from build123d import *

# Parameters (mm, degrees)
SKETCH_1_R          = 1.6
SKETCH_1_R_2        = 3
EXTRUDE_1_DEPTH     = 4
SKETCH_4_R          = 5.25
CUT_EXTRUDE_3_DEPTH = 38.854986461


with BuildPart() as part:
    # 草图1 → 凸台-拉伸1 (new body)
    with BuildSketch(Plane.XY):
        with BuildLine():
            Line((1.833333333, 10.846146269), (31, 5.916079783))
            ThreePointArc((31, 5.916079783), (36, 0), (31, -5.916079783))
            Line((31, -5.916079783), (1.833333333, -10.846146269))
            ThreePointArc((1.833333333, -10.846146269), (-11, 0), (1.833333333, 10.846146269))
        make_face()
        with Locations((0, 7)):
            Circle(SKETCH_1_R, mode=Mode.SUBTRACT)
        with Locations((-7, 0)):
            Circle(SKETCH_1_R, mode=Mode.SUBTRACT)
        with Locations((0, -7)):
            Circle(SKETCH_1_R, mode=Mode.SUBTRACT)
        with Locations((7, 0)):
            Circle(SKETCH_1_R, mode=Mode.SUBTRACT)
        with Locations((30, 0)):
            Circle(SKETCH_1_R_2, mode=Mode.SUBTRACT)
    extrude(amount=EXTRUDE_1_DEPTH)

    # 草图4 → 切除-拉伸3 (cut, through all)
    with BuildSketch(Plane.XY.offset(4)):
        Circle(SKETCH_4_R)
    extrude(amount=-CUT_EXTRUDE_3_DEPTH, mode=Mode.SUBTRACT)


solid = part.part
Design review of the part built by this model. Coordinates are the model's own, in mm. Round coordinates to 2 decimals unless told otherwise and drop trailing zeros. Order: outer loops, then holes, each group sorted by start corner. A loop starts at its lowest first (then second) coordinate and runs counter-clockwise, first axis right, second up. Notation, with made-up numbers: M -32.75,11 L 1.25,11 A15 cw 1.25,31 Z; hole C -36.75,-22 d5. An arc over 180 degrees is marked long. Answer as CSV lines item,"result". Start each with the question number.
1) Add section A-A (z = 3). Give the boundary of the cut face in (x, y), then the cut area to 3 significant figures.
2) Wall thickness on line 1 along Y through (x, z) = (0, 1.5); line 2 along X through (y, z) = (-1.75, 2.5); line 3 along Y through (x, z) = (7, 1.3): over which ranges is each line inside the solid? List them lowest first. Write a range as [from, to].
3) The part is to be moulded in two halves that separate along Y. For faces 1 (the face through (5.4, 0.07, 1.97)), 2 (the face through (13, 0, 0)), 3 (the face through (-11, 0, 2)), 4 (the face through (5, 1.6, 2)), say which applies: +Y half, -Y half, draft (parallel to the pull), parting line (faces both ways), or undercut.
4) Add section C-C (y = 7). Give the boundary of the cut face in (x, z), then the cut area to 3 significant figures.
5) For pin 1 Ø2 at (y, z) = (-5, 2.5) entering from +X; pin 2 Ø2 at (y, z) = (-6.5, 2) entering from +X, all flat-tipped, find the tip position at first contact; note any pin that passes through.
6) Add section B-B (x = 4.5). Give the boundary of the cut face in (y, z).
Resolved:
1,outline,"M 1.83,-10.85 L 31,-5.92 A6 ccw 31,5.92 L 1.83,10.85 A11 ccw long Z; hole C -7,0 d3.2; hole C 0,0 d10.5; hole C 0,-7 d3.2; hole C 0,7 d3.2; hole C 7,0 d3.2; hole C 30,0 d6"
1,area,"617 mm^2"
2,line 1,"[-11, -8.6], [-5.4, -5.25], [5.25, 5.4], [8.6, 11]"
2,line 2,"[-10.86, -4.95], [4.95, 27.56], [32.44, 35.74]"
2,line 3,"[-9.97, -1.6], [1.6, 9.97]"
3,face 1,"undercut"
3,face 2,"draft"
3,face 3,"parting line"
3,face 4,"undercut"
4,outline,"M -8.49,0 L -1.6,0 L -1.6,4 L -8.49,4 Z; M 1.6,0 L 24.59,0 L 24.59,4 L 1.6,4 Z"
4,area,"119 mm^2"
5,pin 1,"x = 34.47"
5,pin 2,"x = 32.4"
6,outline,"M -10.4,0 L -2.7,0 L -2.7,4 L -10.4,4 Z; M 2.7,0 L 10.4,0 L 10.4,4 L 2.7,4 Z"
